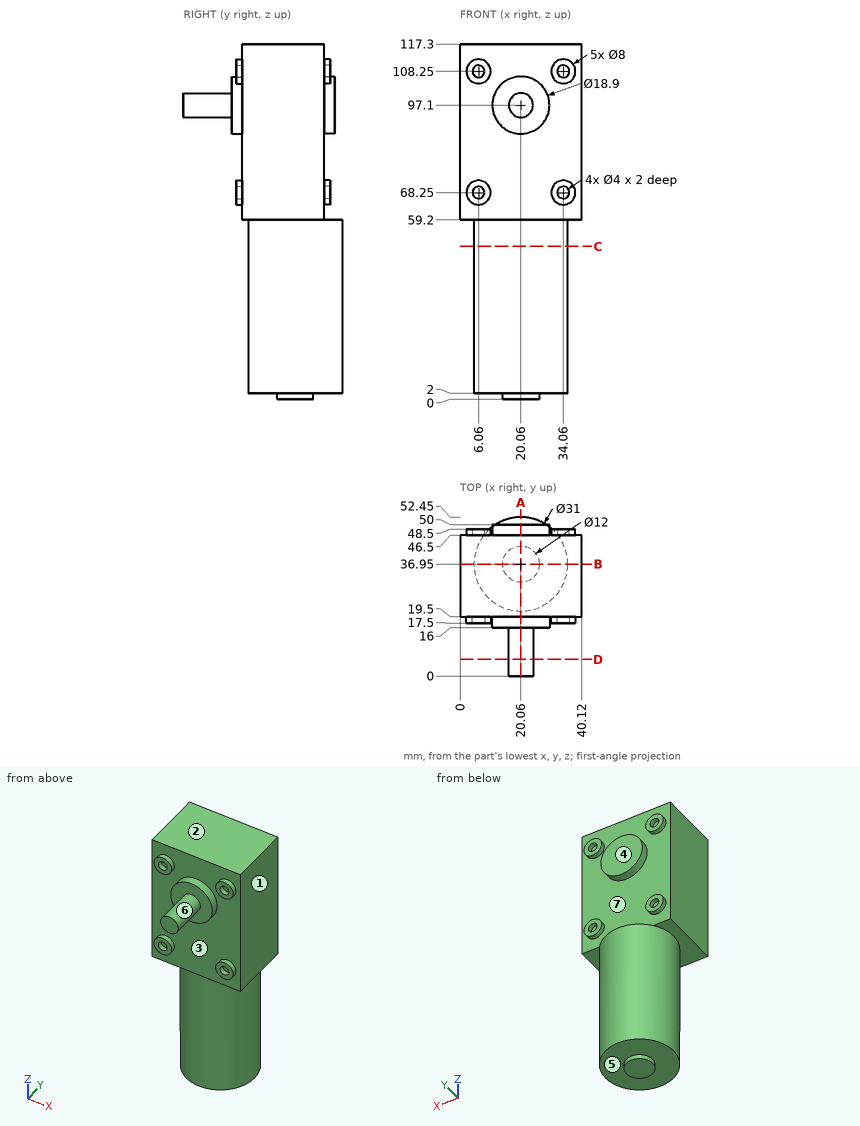
Print and shaded views of the part. All mm, measured from the part's lowest x, y and z. A direction names the side the tool comes from. Coordinates: 2 decimals unless noted, no trailing zeros. Write each loop counter-clockwise with the first axis right and the second up, starting at its lowest first coordinate (ties: lowest second). Pieces come first, ordered by that corner, then holes. Notation, with made-up numbers: M -20.5,68.5 L 21.5,68.5 A24 ccw 21.5,95.5 Z; hole C 81.5,65.5 d10. An arc over 180 degrees is marked long. Return JSON: item names as keys, results as strings.
1. Flat gauge pins, fed straight in: pin 1 Ø2 at (y, z) = (30, 38) entering from -X; pin 2 Ø3 at (x, z) = (33.5, 69) entering from -Y; pin 3 Ø2.5 at (x, z) = (6.06, 108.25) entering from +Y. Where does each tip first touch, or does it go through?
Determined:
{"pin 1": "x = 5.75", "pin 2": "y = 17.5", "pin 3": "y = 46.5"}
2. Saw through at B-B, the plane y = 36.95. Write the cut outline in (x, z).
Determined:
{"outline": "M 0,59.2 L 4.56,59.2 L 4.56,2 L 14.06,2 L 14.06,0 L 26.06,0 L 26.06,2 L 35.56,2 L 35.56,59.2 L 40.12,59.2 L 40.12,117.3 L 0,117.3 Z"}
3. Saw through at D-D, the plane y = 5.5. Write the cut outline in (x, z).
Determined:
{"outline": "C 20.06,97.1 d8"}
4. Pull direction Z, two halves, no side cores. Call the marked faces 1, 2 and 3: pulls with the +Z half, pulls with the -Z half, needs draft (parallel to the pull), parting line crosses it, or undercut.
Determined:
{"face 1": "needs draft", "face 2": "pulls with the +Z half", "face 3": "undercut"}
5. Probe L1, parallel to Z at x = 34.06, y = 18.4; L2, parallel to X at y = 47, z = 108; L3, parallel to Z at x = 8.5, y = 47. List the from-to ranges inside material, lowest first.
Determined:
{"L1": "64.25 to 66.25, 70.25 to 72.25, 104.25 to 106.25, 110.25 to 112.25", "L2": "2.07 to 4.08, 8.04 to 10.05, 30.07 to 32.08, 36.04 to 38.05", "L3": "2 to 59.2, 65.08 to 71.42, 105.08 to 111.42"}
6. Saw through at C-C, the plane z = 50.5. Write the cut outline in (x, y), then the cut area to 3 significant figures.
Determined:
{"outline": "C 20.06,36.95 d31", "area": "755 mm²"}
7. Saw through at A-A, the plane x = 20.06. Write the cut outline in (y, z), then the cut area to 3 significant figures.
Determined:
{"outline": "M 0,93.1 L 16,93.1 L 16,87.65 L 19.5,87.65 L 19.5,59.2 L 21.45,59.2 L 21.45,2 L 30.95,2 L 30.95,0 L 42.95,0 L 42.95,2 L 52.45,2 L 52.45,59.2 L 46.5,59.2 L 46.5,87.65 L 50,87.65 L 50,106.55 L 46.5,106.55 L 46.5,117.3 L 19.5,117.3 L 19.5,106.55 L 16,106.55 L 16,101.1 L 0,101.1 Z", "area": "3,630 mm²"}
8. 3-axis set-ups, long thin cutter, end or side, ignore diameter. For the marked faces 4, 5, 6 and 7: which of +Z, -Z, +X, -X, +Y, -Y reach the whole face in a straight line?
Determined:
{"face 4": "+Z, +X, -X, +Y", "face 5": "-Z", "face 6": "-Y", "face 7": "+Y"}
